Read the model definition and answer for the solid it produces. Units are mm, in the model's axes. Coordinates: 2 decimals unless noted, no trailing zeros. Write each loop counter-clockwise with the first axis right and the second up, starting at its lowest first coordinate (ties: lowest second). Pieces come first, ordered by that corner, then holes. Notation, with made-up numbers: M 15,-28 L 46,-28 A11 ccw 46,-15 Z; hole C -15,-16 d4. An arc over 180 degrees is marked long. Use a Markdown table: item, result. Add a question column.
from build123d import *

# Parameters (mm, degrees)
SKETCH1_R           = 32.27
SKETCH1_R_2         = 25
BOSS_EXTRUDE1_DEPTH = 6.74
CHAMFER1_SIZE       = 0.635
CHAMFER2_SIZE       = 0.635


with BuildPart() as part:
    # Sketch1 → Boss-Extrude1 (new body)
    with BuildSketch(Plane(origin=(0, 0, 0), x_dir=(0, 0, -1), z_dir=(1, 0, 0))):
        Circle(SKETCH1_R)
        Circle(SKETCH1_R_2, mode=Mode.SUBTRACT)
    extrude(amount=BOSS_EXTRUDE1_DEPTH)

    # Chamfer1
    chamfer1_edges = [part.edges().sort_by_distance(p)[0] for p in [
        (0, 0, 32.27),
        (6.74, 0, 32.27),
    ]]
    chamfer(chamfer1_edges, length=CHAMFER1_SIZE)

    # Chamfer2
    chamfer2_edges = [part.edges().sort_by_distance(p)[0] for p in [
        (0, 0, 25),
        (6.74, 0, 25),
    ]]
    chamfer(chamfer2_edges, length=CHAMFER2_SIZE)


solid = part.part
Item 1: Consider probe 1 along Y at (x, z) = (1, 0); probe 2 along Z at (x, y) = (4, -0.5) (3 decimals); probe 3 along Z at (x, y) = (3.5, -9.5). Determine where each line is inside the solid, lowest interval first.
Item 2: Determine the mould class of faces 1 (the flat face through (0, 26, 0)), 2 (the cylindrical face through (3.3, -31.5, 7)), 3 (the cylindrical face through (3.332, 7.509, -23.846)) for opening direction Z: pulls with the +Z half, pulls with the -Z half, needs draft (parallel to the pull), parting line crosses it, or undercut.
Item 3: Find section C-C on x = 4.25. Give the vertices of the cut face in (y, z), then the cut area to 3 significant figures.
Item 4: Find section A-A on y = 0. Give the vertices of the cut face in (x, z) (3 decimals), then the cut area to 3 significant figures.
Item 5: Each of these flat-tipped pins is pushed along its axis until it touches: pin 1 (2 mm diameter, centred on x = 6, z = -24, fed in from +Y); pin 2 (1.5 mm diameter, centred on x = 5, z = 20, fed in from +Y); pin 3 (1.5 mm diameter, centred on x = 3, y = 0.5, fed in from +Z); pin 4 (1 mm diameter, centred on x = 1, z = 12.5, fed in from +Y). Where does it stop, or does it pass through?
Geometry says:
| question | item | result |
|---|---|---|
| 1 | probe 1 | y = -32.27 to -25, 25 to 32.27 |
| 1 | probe 2 | z = -32.266 to -24.995, 24.995 to 32.266 |
| 1 | probe 3 | z = -30.84 to -23.12, 23.12 to 30.84 |
| 2 | face 1 | needs draft |
| 2 | face 2 | parting line crosses it |
| 2 | face 3 | undercut |
| 3 | outline | C 0,0 d64.54; hole C 0,0 d50 |
| 3 | area | 1,310 mm2 |
| 4 | outline | M 0,-31.635 L 0.635,-32.27 L 6.105,-32.27 L 6.74,-31.635 L 6.74,-25.635 L 6.105,-25 L 0.635,-25 L 0,-25.635 Z; M 0,25.635 L 0.635,25 L 6.105,25 L 6.74,25.635 L 6.74,31.635 L 6.105,32.27 L 0.635,32.27 L 0,31.635 Z |
| 4 | area | 96.4 mm2 |
| 5 | pin 1 | stops at y = 22.64 |
| 5 | pin 2 | stops at y = 25.9 |
| 5 | pin 3 | stops at z = 32.27 |
| 5 | pin 4 | stops at y = 29.96 |
